Geometry check sheet. Reference: the model listing, model coordinates, mm. Face numbers are marked on the shaded views. Round coordinates to 2 decimals unless told otherwise and drop trailing zeros. Write each loop counter-clockwise with the first axis right and the second up, starting at its lowest first coordinate (ties: lowest second). Pieces come first, ordered by that corner, then holes. Notation, with made-up numbers: (37.5, -25) - (68.5, -25) arc R19 ccw to (68.5, -4) - close; hole circle Ø8 at (-17.5, -6.5). An arc over 180 degrees is marked (long way). Return JSON: item names as keys, results as strings.
```python
from build123d import *

# Parameters (mm, degrees)
F0_R     = 9.525
F1_DEPTH = 7.15
F2_R     = 0.508
F3_DEPTH = 5


with BuildPart() as f1:
    # F0 (on Front) → F1 (new body, symmetric)
    with BuildSketch(Plane.XZ):
        with BuildLine():
            ThreePointArc((22.25, 22.25), (0, 44.5), (-22.25, 22.25))
            Line((-22.25, 22.25), (-22.25, 0))
            Line((-22.25, 0), (22.25, 0))
            Line((22.25, 0), (22.25, 22.25))
        make_face()
        with Locations((0, 22.25)):
            Circle(F0_R, mode=Mode.SUBTRACT)
    extrude(amount=F1_DEPTH, both=True)

    # F2 (on face) → F3 (join)
    with BuildSketch(Plane(origin=(0, 0, 0), x_dir=(1, 0, 0), z_dir=(0, 0, -1))):
        with Locations((-17.78, 5.08)):
            Circle(F2_R)
        with Locations((17.78, 5.08)):
            Circle(F2_R)
        with Locations((0, -5.08)):
            Circle(F2_R)
    extrude(amount=F3_DEPTH)


solid = f1.part
```
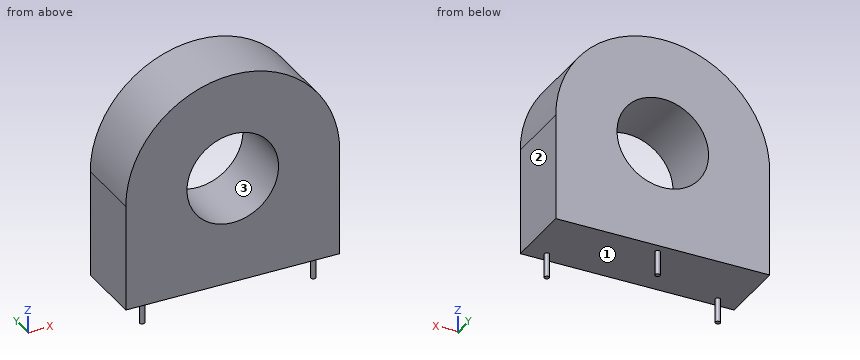
(1) Section check D-D, the plane z = 38.5. Enter the section's corners in (x, y).
Response values:
{"outline": "(-15.2, -7.15) - (15.2, -7.15) - (15.2, 7.15) - (-15.2, 7.15) - close"}
(2) Release check for a two-part mould opening along Z. For the marked faces 1, 2 and 3 record: pulls with the +Z half, pulls with the -Z half, needs draft (parallel to the pull), parting line crosses it, or undercut.
Response values:
{"face 1": "pulls with the -Z half", "face 2": "needs draft", "face 3": "undercut"}
(3) Gauge pin test, flat ends, axial feed: pin 1 (3 mm diameter, centred on y = -3.5, z = 26.5, fed in from +X); pin 2 (2 mm diameter, centred on y = -3, z = 32, fed in from -X); pin 3 (2 mm diameter, centred on x = -3, y = -1.5, fed in from +Z). Record the tip position at first contact, or that the pin passes through.
Response values:
{"pin 1": "stops at x = 22.08", "pin 2": "stops at x = -20.46", "pin 3": "stops at z = 44.41"}
(4) Section check C-C, the plane z = 31. Enter the section's corners in (x, y), plus the area to 3 significant figures.
Response values:
{"outline": "(-20.46, -7.15) - (-3.76, -7.15) - (-3.76, 7.15) - (-20.46, 7.15) - close; (3.76, -7.15) - (20.46, -7.15) - (20.46, 7.15) - (3.76, 7.15) - close", "area": "477 mm^2"}
(5) Material ranges on line 1 along Z through (x, y) = (0, 0) (3 decimals); line 2 along X through (y, z) = (3.25, 18); line 3 along X through (y, z) = (-6.5, 29.5), recorded low to high. Write a range as [from, to].
Response values:
{"line 1": "z = [0, 12.725], [31.775, 44.5]", "line 2": "x = [-22.25, -8.52], [8.52, 22.25]", "line 3": "x = [-21.04, -6.18], [6.18, 21.04]"}
(6) Section check A-A, the plane y = -3.25. Enter the section's corners in (x, z) (3 decimals).
Response values:
{"outline": "(-22.25, 0) - (22.25, 0) - (22.25, 22.25) arc R22.25 ccw to (-22.25, 22.25) - close; hole circle Ø19.05 at (0, 22.25)"}
(7) Section check B-B, the plane x = -5.5. Enter the section's corners in (y, z).
Response values:
{"outline": "(-7.15, 0) - (7.15, 0) - (7.15, 14.47) - (-7.15, 14.47) - close; (-7.15, 30.03) - (7.15, 30.03) - (7.15, 43.81) - (-7.15, 43.81) - close"}
